Check sheet for the drawn part. Datum: minimum x, y, z corner. Units: mm. A direction names the side the tool comes from. Give positions to 0.01 mm unless a question says otherwise; leave off trailing zeros. Loops run counter-clockwise (first coordinate to the right, second up) from the corner with the lowest first, then second, coordinate; pieces in that order, holes last. Notation, with made-up numbers: M 11.5,71.25 L 24.5,71.25 A32 ccw 24.5,108.25 Z; hole C 72.25,25 d6. An arc over 180 degrees is marked long. Write each question's results on one line, items separated by ' | '. Start each with the question number.
1. Tool access check on the marked faces 1, 2 and 3. Record the directions out of +Z, -Z, +X, -X, +Y, -Y that give a thin tool (end or side, any length) a straight path to the whole face; none if there is none.
2. Sectioned sample at B-B on y = 10.5. Record the cut outline in (x, z).
3. Sectioned sample at C-C on z = 0.75. Record the cut outline in (x, y).
4. Material ranges on line 1 along X through (y, z) = (20, 7); line 2 along Y through (x, z) = (16.75, 2.5); line 3 along X through (y, z) = (3.25, 4), recorded low to high.
5. Go/stop test with flat-tipped pins: pin 1 (3 mm diameter, centred on x = 18, z = 6, fed in from +Y); pin 2 (4 mm diameter, centred on y = 15, z = 4, fed in from -X); pin 3 (3 mm diameter, centred on y = 21.5, z = 6.5, fed in from -X). Record where each tip stops, or that it passes through.
6. Sectioned sample at A-A on x = 21.75. Record the cut outline in (y, z), and give its area (3 significant figures).
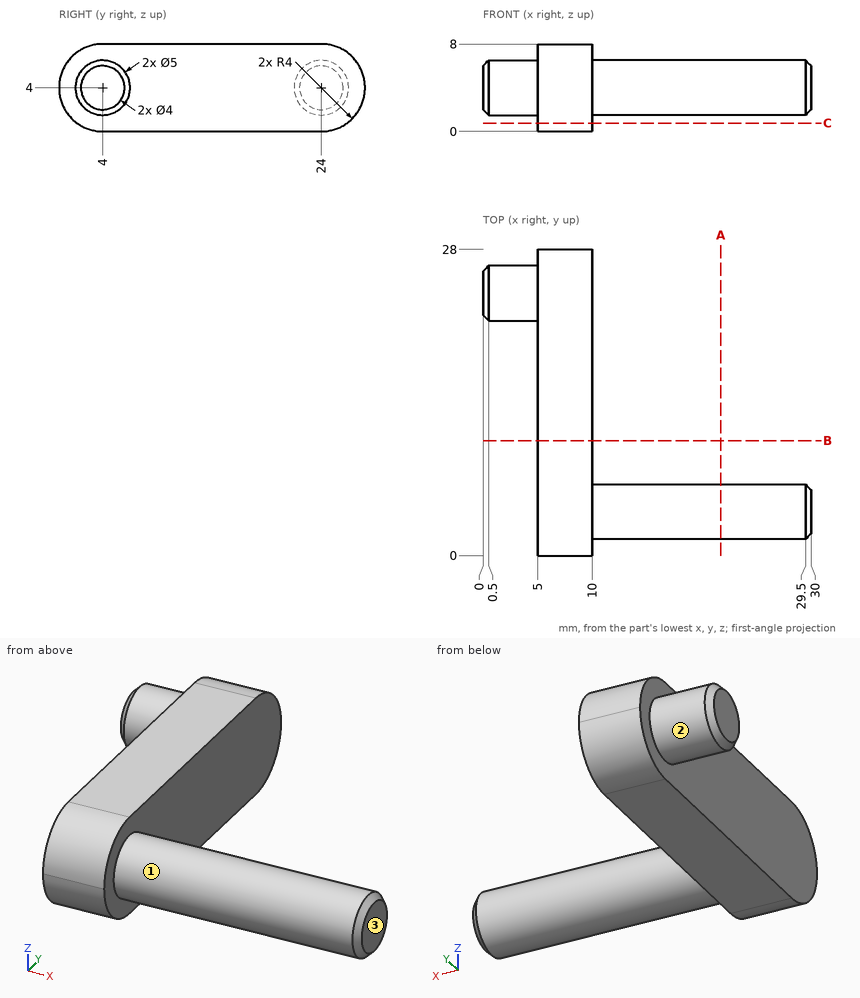
Output values:
1) face 1: +X | face 2: -X | face 3: +Z, -Z, +X, +Y, -Y
2) outline: M 5,0 L 10,0 L 10,8 L 5,8 Z
3) outline: M 5,1.67 L 10,1.67 L 10,26.33 L 5,26.33 Z
4) line 1: 5 to 10 | line 2: 2 to 6 | line 3: 5 to 30
5) pin 1: y = 6.45 | pin 2: x = 5 | pin 3: x = 0.04
6) outline: C 4,4 d5 | area: 19.6 mm2
